```python
from build123d import *

# Parameters (mm, degrees)
BOSS_EXTRU_1_DEPTH       = 20
ESQUISSE2_R              = 7
ENL_V_MAT_EXTRU_1_DEPTH  = 36.665109
CHANFREIN1_SIZE          = 1
ENL_V_MAT_EXTRU_3_DEPTH  = 36.665109
CONG_1_R                 = 20
ENL_V_MAT_EXTRU_4_DEPTH  = 36.665109168
CONG_2_R                 = 3
CONG_3_R                 = 2
CONG_2_OF_SYM_TRIE1_R    = 3
CONG_3_OF_SYM_TRIE1_R    = 2
ESQUISSE7_W              = 3
ESQUISSE7_H              = 19.363772413
ENL_V_MAT_EXTRU_5_DEPTH  = 2
ESQUISSE8_R              = 2
ENL_V_MAT_EXTRU_6_DEPTH  = 36.665109168
ENL_V_MAT_EXTRU_7_DEPTH  = 2
ENL_V_MAT_EXTRU_8_DEPTH  = 1
ENL_V_MAT_EXTRU_9_DEPTH  = 2
ENL_V_MAT_EXTRU_10_DEPTH = 0.5


with BuildPart() as part:
    # Esquisse1 → Boss.-Extru.1 (new body)
    with BuildSketch(Plane.XY):
        with BuildLine():
            Line((-14, -12), (-14, 12))
            ThreePointArc((-14, 12), (0, 26), (14, 12))
            Line((14, 12), (14, -12))
            ThreePointArc((14, -12), (0, -26), (-14, -12))
        make_face()
    extrude(amount=BOSS_EXTRU_1_DEPTH)

    # Esquisse2 → Enlèv. mat.-Extru.1 (cut, through all)
    with BuildSketch(Plane.XY.offset(20)):
        with Locations((0, 12)):
            Circle(ESQUISSE2_R)
        with Locations((0, -12)):
            Circle(ESQUISSE2_R)
    extrude(amount=-ENL_V_MAT_EXTRU_1_DEPTH, mode=Mode.SUBTRACT)

    # Chanfrein1
    chanfrein1_edges = [part.edges().sort_by_distance(p)[0] for p in [
        (-7, 12, 20),
        (-7, -12, 20),
    ]]
    chamfer(chanfrein1_edges, length=CHANFREIN1_SIZE)

    # Esquisse3 → Enlèv. mat.-Extru.3 (cut, through all)
    with BuildSketch(Plane.XY.offset(20)):
        with BuildLine():
            Line((-14, 12), (-14, -12))
            ThreePointArc((-14, -12), (-12.185143325, -5.106359297), (-7.211102551, 0))
            ThreePointArc((-7.211102551, 0), (-12.185143325, 5.106359297), (-14, 12))
        make_face()
        with BuildLine():
            Line((14, -12), (14, 12))
            ThreePointArc((14, 12), (12.185143325, 5.106359297), (7.211102551, 0))
            ThreePointArc((7.211102551, 0), (12.185143325, -5.106359297), (14, -12))
        make_face()
    extrude(amount=-ENL_V_MAT_EXTRU_3_DEPTH, mode=Mode.SUBTRACT)

    # Congé1
    cong_1_edges = [part.edges().sort_by_distance(p)[0] for p in [
        (7.211102551, 0, 10),
        (-7.211102551, 0, 10),
    ]]
    fillet(cong_1_edges, radius=CONG_1_R)

    # Esquisse6 → Enlèv. mat.-Extru.4 (cut, through all)
    with BuildSketch(Plane.XY.offset(20)):
        Polygon((-12.985436878, 6.75), (-11.773762969, 6.536349198), (-8, 0), (-11.773762969, -6.536349198), (-12.985436878, -6.75), align=None)
    enl_v_mat_extru_4 = extrude(amount=-ENL_V_MAT_EXTRU_4_DEPTH, mode=Mode.SUBTRACT)

    # Congé2
    cong_2_edges = [part.edges().sort_by_distance(p)[0] for p in [
        (-8, 0, 10),
    ]]
    fillet(cong_2_edges, radius=CONG_2_R)

    # Congé3
    cong_3_edges = [part.edges().sort_by_distance(p)[0] for p in [
        (-11.773762969, 6.536349198, 10),
        (-11.773762969, -6.536349198, 10),
    ]]
    fillet(cong_3_edges, radius=CONG_3_R)

    # Symétrie1: Enlèv. mat.-Extru.4 across plane
    add(enl_v_mat_extru_4.mirror(Plane(origin=(0, 0, 0), x_dir=(0, 0, 1), z_dir=(1, 0, 0))), mode=Mode.SUBTRACT)

    # Congé2 of Symétrie1
    cong_2_of_sym_trie1_edges = [part.edges().sort_by_distance(p)[0] for p in [
        (8, 0, 10),
    ]]
    fillet(cong_2_of_sym_trie1_edges, radius=CONG_2_OF_SYM_TRIE1_R)

    # Congé3 of Symétrie1
    cong_3_of_sym_trie1_edges = [part.edges().sort_by_distance(p)[0] for p in [
        (11.773762969, 6.536349198, 10),
        (11.773762969, -6.536349198, 10),
    ]]
    fillet(cong_3_of_sym_trie1_edges, radius=CONG_3_OF_SYM_TRIE1_R)

    # Esquisse7 → Enlèv. mat.-Extru.5 (cut)
    with BuildSketch(Plane.XY.offset(20)):
        with Locations((4, -0.240073956)):
            Rectangle(ESQUISSE7_W, ESQUISSE7_H)
    extrude(amount=-ENL_V_MAT_EXTRU_5_DEPTH, mode=Mode.SUBTRACT)

    # Esquisse8 → Enlèv. mat.-Extru.6 (cut, through all)
    with BuildSketch(Plane.XY.offset(20)):
        with Locations((-4.25, 16)):
            Circle(ESQUISSE8_R)
        with Locations((-4.25, -16)):
            Circle(ESQUISSE8_R)
    extrude(amount=-ENL_V_MAT_EXTRU_6_DEPTH, mode=Mode.SUBTRACT)

    # Esquisse9 → Enlèv. mat.-Extru.7 (cut)
    with BuildSketch(Plane.XY.offset(20)):
        with BuildLine():
            Line((-12.985436878, 6.75), (-2.638783858, 2.938351237))
            ThreePointArc((-2.638783858, 2.938351237), (-2, 1.824431263), (-2.984467175, 1))
            Line((-2.984467175, 1), (-6.5, 1))
            ThreePointArc((-6.5, 1), (-7.5, 0), (-6.5, -1))
            Line((-6.5, -1), (-2.984467175, -1))
            ThreePointArc((-2.984467175, -1), (-2, -1.824431263), (-2.638783858, -2.938351237))
            Line((-2.638783858, -2.938351237), (-12.985436878, -6.75))
            Line((-12.985436878, -6.75), (-12.985436878, 6.75))
        make_face()
    extrude(amount=-ENL_V_MAT_EXTRU_7_DEPTH, mode=Mode.SUBTRACT)

    # Esquisse10 → Enlèv. mat.-Extru.8 (cut)
    with BuildSketch(Plane(origin=(0, 0, 0), x_dir=(-1, 0, 0), z_dir=(0, 0, -1))):
        Polygon((-14.880645038, 4.022009348), (-5.050820507, 10.904926585), (-2.756514761, 7.628318408), (-12.586339293, 0.745401171), align=None)
        Polygon((14.104417015, 2.702110502), (8.18518219, 6.119582321), (9.18518219, 7.851633128), (15.104417015, 4.434161309), align=None)
    enl_v_mat_extru_8 = extrude(amount=-ENL_V_MAT_EXTRU_8_DEPTH, mode=Mode.SUBTRACT)

    # Symétrie2: Enlèv. mat.-Extru.8 across plane
    add(enl_v_mat_extru_8.mirror(Plane.ZX), mode=Mode.SUBTRACT)

    # Esquisse11 → Enlèv. mat.-Extru.9 (cut)
    with BuildSketch(Plane(origin=(0, 0, 0), x_dir=(-1, 0, 0), z_dir=(0, 0, -1))):
        with BuildLine():
            Line((-9.821287991, 18.876939886), (-11.46812862, 20.030070109))
            Line((-11.46812862, 20.030070109), (-13.322410066, 19.286515908))
            Line((-13.322410066, 19.286515908), (-12.922465041, 17.386083667))
            Line((-12.922465041, 17.386083667), (-11.5420173, 16.419483753))
            ThreePointArc((-11.5420173, 16.419483753), (-8.998687611, 15.827772592), (-6.753604006, 17.161282102))
            ThreePointArc((-6.753604006, 17.161282102), (7.619740739, 15.766902052), (0, 3.5))
            ThreePointArc((0, 3.5), (-2.474873734, 2.474873734), (-3.5, 0))
            Line((-3.5, 0), (-0.5, 0))
            ThreePointArc((-0.5, 0), (-0.353553391, 0.353553391), (0, 0.5))
            ThreePointArc((0, 0.5), (10.309061, 17.096396894), (-9.137228949, 18.982911079))
            ThreePointArc((-9.137228949, 18.982911079), (-9.457955178, 18.79240972), (-9.821287991, 18.876939886))
        make_face()
    enl_v_mat_extru_9 = extrude(amount=-ENL_V_MAT_EXTRU_9_DEPTH, mode=Mode.SUBTRACT)

    # Esquisse12 → Enlèv. mat.-Extru.10 (cut)
    with BuildSketch(Plane(origin=(0, 0, 1), x_dir=(-1, 0, 0), z_dir=(0, 0, -1))):
        Polygon((-11.722201386, 6.233575403), (-6.642191838, 9.790636383), (-4.347886092, 6.514028206), (-9.626796974, 2.817695012), align=None)
        Polygon((-9.626796974, -2.817695012), (-4.347886092, -6.514028206), (-6.642191838, -9.790636383), (-11.722201386, -6.233575403), align=None)
    extrude(amount=-ENL_V_MAT_EXTRU_10_DEPTH, mode=Mode.SUBTRACT)

    # Symétrie3: Enlèv. mat.-Extru.9 across plane
    add(enl_v_mat_extru_9.mirror(Plane.ZX), mode=Mode.SUBTRACT)


solid = part.part
```
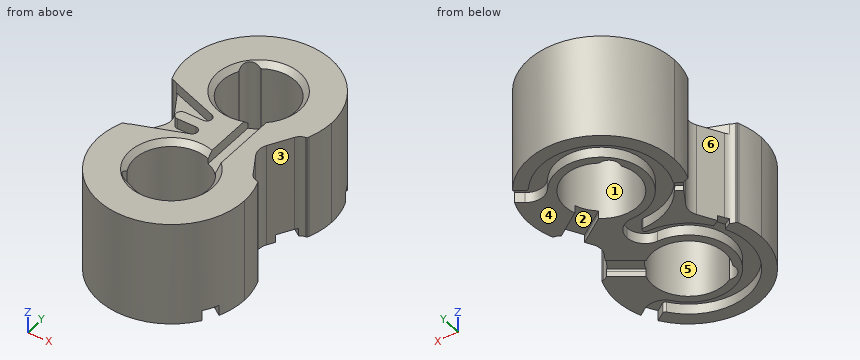
Can you work these out from the model? Positions are in its coordinate system, mm. Face numbers are marked on the shaded views. A direction names the side the tool comes from. Round coordinates to 2 decimals unless told otherwise and drop trailing zeros. Order: outer loops, then holes, each group sorted by start corner. A loop starts at its lowest first (then second) coordinate and runs counter-clockwise, first axis right, second up. Notation, with made-up numbers: (6, -15.75) -> (43, -15.75) arc R26 ccw to (43, 17.25) -> close; hole circle Ø2 at (-21.75, 56). An arc over 180 degrees is marked (long way). Return JSON: item names as keys, results as strings. Group by question number.
1. If we section it at B-B, the plane z = 9: Count the separate pieces of the cut face and the enclosed holes in it, then the cut area to 3 significant figures.
2. Will these pins go through, and if not, where does the flat tip stop? pin 1 (2 mm diameter, centred on x = 8, y = -6, fed in from -Z); pin 2 (2 mm diameter, centred on x = 11, z = 15, fed in from -Y); pin 3 (1 mm diameter, centred on x = -4.5, z = 18.5, fed in from -Y).
3. I need wall thicknesses on line 1 (X direction, y = -12, z = 1.1); line 2 (X direction, y = -12, z = 5.25); line 3 (X direction, y = 13, z = 1). Which ranges of each line are inside material? Lowest first, please. Write a range as [from, to].
4. If we section it at A-A, the plane x = 10.5: Write out the boundary of the cut face in (y, z).
5. Which directions (+Z, -Z, +X, -X, +Y, -Y) give clear straight access to the entire face, cutting with the end or side of a thin tool? Please do the marked faces 1, 2 and 3.
6. We'd pull the mould along X, two halves only. Please class the marked faces 4, 5 and 6: released by +X, released by -X, zero draft, split by the parting line, or undercut.
Output values:
{
 "1": {"separate pieces": "1", "enclosed holes": "2", "area": "861 mm²"},
 "2": {"pin 1": "z = 1.5", "pin 2": "y = -21.8", "pin 3": "y = -25.42"},
 "3": {"line 1": "[-14, -11.5], [-8.5, -7], [7, 14]", "line 2": "[-14, -7], [7, 14]", "line 3": "[-13.96, -11.46], [-8.44, -6.93], [6.93, 13.96]"},
 "4": {"outline": "(-21.26, 0) -> (-19.35, 0) -> (-19.35, 2) -> (-15.92, 2) -> (-15.92, 0) -> (-7.09, 0) -> (-7.09, 1.5) -> (-4.33, 1.5) -> (-4.33, 20) -> (-21.26, 20) -> close; (4.33, 1.5) -> (7.09, 1.5) -> (7.09, 0) -> (15.92, 0) -> (15.92, 2) -> (19.35, 2) -> (19.35, 0) -> (21.26, 0) -> (21.26, 20) -> (4.33, 20) -> close"},
 "5": {"face 1": "+Z, -Z", "face 2": "-Z", "face 3": "+Z, -Z, +X"},
 "6": {"face 4": "zero draft", "face 5": "undercut", "face 6": "released by -X"}
}
